Check sheet for the modelled part. Datum: model origin and axes. Units: mm. A direction names the side the tool comes from. Round coordinates to 2 decimals unless told otherwise and drop trailing zeros. Order: outer loops, then holes, each group sorted by start corner. A loop starts at its lowest first (then second) coordinate and runs counter-clockwise, first axis right, second up.
Q1. Cross-section at B-B on z = 15.5. Record the cut outline in (x, y).
Q2. Mould release check, pull along Y, two halves, no side actions. Record for faces 1 (the cylindrical face through (5.916, -6.627, 26.856)), 2 (the cylindrical face through (6.084, -15.713, 12.248)), 3 (the cylindrical face through (6.084, -19.248, 12.287)), 4 (the flat face through (6, 25, -5)): +Y half, -Y half, draft (parallel to the pull), parting line (faces both ways), or undercut.
Q3. Set-up check for faces 5 (the flat face through (6, 12, 25)), 6 (the flat face through (6, -10, 0)), 7 (the flat face through (6, 0, 10)): record each of +Z, -Z, +X, -X, +Y, -Y from which the full face is reachable in a straight line by a thin tool's end or side.
Q4. Cross-section at D-D on y = 19. Record the cut outline in (x, z), then the cut area to 3 significant figures.
Q5. Depth check by flat-ended pin: P1, Ø1.5, axis at y = -3, z = 18, coming from the -X side; P2, Ø4, axis at x = 1.5, y = 6, coming from the +Z side; P3, Ø6, axis at x = 3, y = 6.5, coming from the -Z side; P4, Ø5.5, axis at x = 6, y = -10.5, coming from the +Z side. Enter the tip coordinate at first touch or a pass-through.
Q6. Scan lines: probe 1 along Y at (x, z) = (3, 15.5); probe 2 along Z at (x, y) = (3.75, 12); probe 3 along Y at (x, z) = (6.25, 4.5). Record each from-to range of solid material in increasing order.
Q7. Cross-section at A-A on z = 9.5. Record the cut outline in (x, y).
from build123d import *

# Parameters (mm, degrees)
F1_DEPTH = 12
F2_R     = 2.49999


# Not quite as in the source:
# - a fillet or chamfer is up to 0.001 mm smaller than in the source, because OpenCascade refuses the exact size


with BuildPart() as f1:
    # F0 (on Right) → F1 (new body)
    with BuildSketch(Plane.YZ):
        Polygon((-20, 0), (0, 0), (0, 20), (-5, 25), (-5, 17.0456439427), (-5, 5), (-15, 5), (-15, 13), (-20, 13), align=None)
        Polygon((-5, 25), (0, 20), (24, 20), (29, 25), (21.0456439427, 25), (2.9543560573, 25), align=None)
        Polygon((29, 25), (24, 20), (24, -5), (29, -5), (29, 17.0456439427), align=None)
        with BuildLine():
            Line((-5, 17.0456439427), (-5, 25))
            Line((-5, 25), (2.9543560573, 25))
            ThreePointArc((2.9543560573, 25), (-6.7426406871, 26.7426406871), (-5, 17.0456439427))
        make_face()
        with BuildLine():
            Line((21.0456439427, 25), (29, 25))
            Line((29, 25), (29, 17.0456439427))
            ThreePointArc((29, 17.0456439427), (30.7426406871, 26.7426406871), (21.0456439427, 25))
        make_face()
    extrude(amount=F1_DEPTH)

    # F2 (radius 2.5 in the source; OpenCascade refuses exactly that, so slightly less here)
    f2_edges = [f1.edges().sort_by_distance(p)[0] for p in [
        (6, -5, 5),
        (6, -15, 5),
        (6, 29, -5),
        (6, -20, 13),
        (6, -15, 13),
    ]]
    fillet(f2_edges, radius=F2_R)


solid = f1.part
Results found:
1. outline: (0, -5) - (12, -5) - (12, 0) - (0, 0) - close; (0, 24) - (12, 24) - (12, 29) - (0, 29) - close
2. face 1: undercut
2. face 2: undercut
2. face 3: -Y half
2. face 4: draft
3. face 5: +Z, +X, -X
3. face 6: -Z, +X, -X, -Y
3. face 7: -Z, +X, -X
4. outline: (0, 20) - (12, 20) - (12, 25) - (0, 25) - close
4. area: 60.0 mm2
5. P1: stops at x = 0
5. P2: stops at z = 25
5. P3: stops at z = 20
5. P4: stops at z = 25.4
6. probe 1: y = -5 to 0, 24 to 29
6. probe 2: z = 20 to 25
6. probe 3: y = -20 to 0, 24 to 29
7. outline: (0, -20) - (12, -20) - (12, -15) - (0, -15) - close; (0, -5) - (12, -5) - (12, 0) - (0, 0) - close; (0, 24) - (12, 24) - (12, 29) - (0, 29) - close
